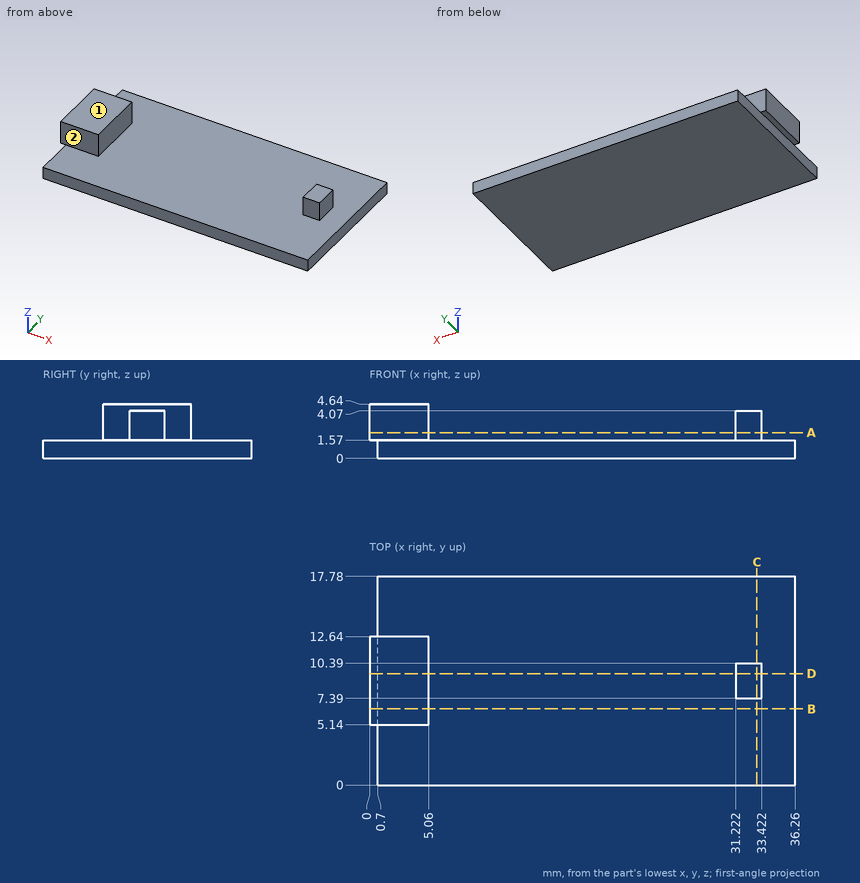
Study the drawing (mm; zero at the part's minimum x, y, z) and answer. A direction names the side the tool comes from. Give positions to 0.01 mm unless a question says otherwise; leave off trailing zeros. Loops run counter-clockwise (first coordinate to the right, second up) from the corner with the lowest first, then second, coordinate; pieces in that order, holes last. Notation, with made-up numbers: M 78.5,74 L 120.5,74 A24 cw 120.5,86 Z; hole C 76.25,-2.75 d6. An arc over 180 degrees is marked long. Use CSV: the item, a comma, the result in double quotes.
1) Find section A-A on z = 2.2. Write down the section's boundary in (x, y).
Answer:
outline,"M 0,5.14 L 5.06,5.14 L 5.06,12.64 L 0,12.64 Z; M 31.22,7.39 L 33.42,7.39 L 33.42,10.39 L 31.22,10.39 Z"
2) Consider L1, parallel to Y at x = 4.5, z = 3.7; L2, parallel to X at y = 10.5, z = 2.9; L3, parallel to X at y = 9.75, z = 3.95. Determine where each line is inside the solid, lowest interval first.
Answer:
L1,"5.14 to 12.64"
L2,"0 to 5.06"
L3,"0 to 5.06, 31.22 to 33.42"
3) Find section D-D on y = 9.5. Write down the section's boundary in (x, z).
Answer:
outline,"M 0,1.57 L 0.7,1.57 L 0.7,0 L 36.26,0 L 36.26,1.57 L 33.42,1.57 L 33.42,4.07 L 31.22,4.07 L 31.22,1.57 L 5.06,1.57 L 5.06,4.64 L 0,4.64 Z"
4) Find section C-C on x = 33. Write down the section's boundary in (y, z).
Answer:
outline,"M 0,0 L 17.78,0 L 17.78,1.57 L 10.39,1.57 L 10.39,4.07 L 7.39,4.07 L 7.39,1.57 L 0,1.57 Z"
5) Given P1, Ø0.7, axis at x = 32.5, y = 8.5, coming from the +Z side; P2, Ø1.5, axis at y = 10.5, z = 3.5, coming from the +X side; P3, Ø4, axis at x = 30, y = 13, coming from the +Z side, each flat-ended and moving along its own axis, determine where each tip first touches the part or whether it passes through.
Answer:
P1,"z = 4.07"
P2,"x = 33.42"
P3,"z = 1.57"
6) Which of the six approach directions +Z, -Z, +X, -X, +Y, -Y give full straight-line access (tool end or side, diameter ignored) to the marked faces 1 and 2?
Answer:
face 1,"+Z, +X, -X, +Y, -Y"
face 2,"+Z, +X, -X, -Y"
7) Find section B-B on y = 6.5. Write down the section's boundary in (x, z).
Answer:
outline,"M 0,1.57 L 0.7,1.57 L 0.7,0 L 36.26,0 L 36.26,1.57 L 5.06,1.57 L 5.06,4.64 L 0,4.64 Z"
